The model under review builds one solid part; all positions refer to its coordinate system, in mm. Face numbers are marked on the shaded views. Coordinates: 2 decimals unless noted, no trailing zeros. Loops run counter-clockwise (first coordinate to the right, second up) from the corner with the lowest first, then second, coordinate; pieces in that order, holes last. Notation, with made-up numbers: M 5,31 L 9,31 A18 ccw 9,49 Z; hole C 70.25,-38.5 d2. An arc over 180 degrees is marked long. Write item = value, one per line. Start each with the question number.
Q1. We need section C-C on y = -91. Give the boundary of the cut face in (x, z).
Q2. Wall thickness on probe 1 along Y at (x, z) = (156, 52.95); probe 2 along Y at (x, z) = (156.5, 54.1); probe 3 along X at (y, z) = (-66.5, 50.75): over which ranges is each line inside the solid? List them lowest first.
Q3. Mouldability with a two-part tool opening along X and no side actions: class the marked faces 1 and 2 as released by +X, released by -X, zero draft, split by the parting line, or undercut.
Q4. We need section D-D on x = 114.5. Give the boundary of the cut face in (y, z).
Q5. We need section B-B on y = -83.5. Give the boundary of the cut face in (x, z).
Q6. We need section A-A on x = 161.5. Give the boundary of the cut face in (y, z), and give its area (3 significant figures).
from build123d import *

# Parameters (mm, degrees)
SKETCH004_W      = 28
SKETCH004_H      = 18
EXTRUDE004_DEPTH = 1.6
EXTRUDE003_DEPTH = 3


with BuildPart() as obj1:
    # Sketch004 → Extrude004 (new body)
    with BuildSketch(Plane.XY):
        with BuildLine():
            Line((89.498192, -57.050084), (174.498192, -57.050084))
            ThreePointArc((182.698192, -65.250084), (180.296468, -59.451808), (174.498192, -57.050084))
            Line((182.698192, -65.250084), (182.698192, -93.250084))
            ThreePointArc((174.498192, -101.450084), (180.296468, -99.04836), (182.698192, -93.250084))
            Line((174.498192, -101.450084), (89.498192, -101.450084))
            ThreePointArc((81.298192, -93.250084), (83.699916, -99.04836), (89.498192, -101.450084))
            Line((81.298192, -93.250084), (81.298192, -65.250084))
            ThreePointArc((89.498192, -57.050084), (83.699916, -59.451808), (81.298192, -65.250084))
        make_face()
        with Locations((151.513474, -79.24515)):
            Rectangle(SKETCH004_W, SKETCH004_H, mode=Mode.SUBTRACT)
    extrude(amount=EXTRUDE004_DEPTH)


with BuildPart() as obj1_1:
    # Extrude004 placement: moved
    add(obj1.part.moved(Location((0, 0, 53))))


with BuildPart() as obj2:
    # Sketch003 → Extrude003 (new body)
    with BuildSketch(Plane.XY):
        with BuildLine():
            Line((89.498192, -57.050084), (174.498192, -57.050084))
            ThreePointArc((182.698192, -65.250084), (180.296468, -59.451808), (174.498192, -57.050084))
            Line((182.698192, -65.250084), (182.698192, -93.250084))
            ThreePointArc((174.498192, -101.450084), (180.296468, -99.04836), (182.698192, -93.250084))
            Line((174.498192, -101.450084), (89.498192, -101.450084))
            ThreePointArc((81.298192, -93.250084), (83.699916, -99.04836), (89.498192, -101.450084))
            Line((81.298192, -93.250084), (81.298192, -65.250084))
            ThreePointArc((89.498192, -57.050084), (83.699916, -59.451808), (81.298192, -65.250084))
        make_face()
        with BuildLine():
            Line((89.498192, -99.850084), (174.498192, -99.850084))
            ThreePointArc((174.498192, -99.850084), (179.165097, -97.916989), (181.098192, -93.250084))
            Line((181.098192, -93.250084), (181.098192, -65.250084))
            ThreePointArc((181.098192, -65.250084), (179.165097, -60.583179), (174.498192, -58.650084))
            Line((174.498192, -58.650084), (89.498192, -58.650084))
            ThreePointArc((89.498192, -58.650084), (84.831287, -60.583179), (82.898192, -65.250084))
            Line((82.898192, -65.250084), (82.898192, -93.250084))
            ThreePointArc((82.898192, -93.250084), (84.831287, -97.916989), (89.498192, -99.850084))
        make_face(mode=Mode.SUBTRACT)
    extrude(amount=EXTRUDE003_DEPTH)


with BuildPart() as obj2_1:
    # Extrude003 placement: moved
    add(obj2.part.moved(Location((0, 0, 50))))

    # Fusion001: union obj1
    add(obj1_1.part)


solid = obj2_1.part
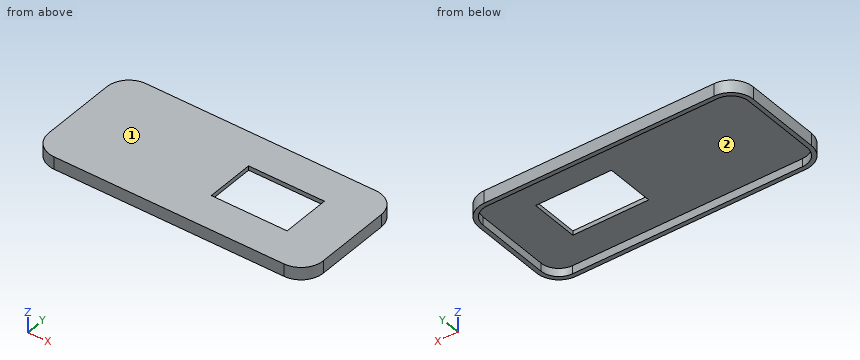
Returned:
q1.outline = M 81.3,50 L 82.9,50 L 82.9,53 L 181.1,53 L 181.1,50 L 182.7,50 L 182.7,54.6 L 81.3,54.6 Z
q2.probe_1 = -101.45 to -99.85, -58.65 to -57.05
q2.probe_2 = -101.45 to -88.25, -70.25 to -57.05
q2.probe_3 = 81.3 to 82.9, 181.1 to 182.7
q3.face_1 = zero draft
q3.face_2 = undercut
q4.outline = M -101.45,50 L -99.85,50 L -99.85,53 L -58.65,53 L -58.65,50 L -57.05,50 L -57.05,54.6 L -101.45,54.6 Z
q5.outline = M 81.3,50 L 82.9,50 L 82.9,53 L 137.51,53 L 137.51,54.6 L 81.3,54.6 Z; M 165.51,53 L 181.1,53 L 181.1,50 L 182.7,50 L 182.7,54.6 L 165.51,54.6 Z
q6.outline = M -101.45,50 L -99.85,50 L -99.85,53 L -88.25,53 L -88.25,54.6 L -101.45,54.6 Z; M -70.25,53 L -58.65,53 L -58.65,50 L -57.05,50 L -57.05,54.6 L -70.25,54.6 Z
q6.area = 51.8 mm^2
